CAD build for the part. Positions are in the model's coordinates, mm. A direction names the side the tool comes from. Give positions to 0.01 mm unless a question says otherwise; leave off trailing zeros. Order: outer loops, then holes, each group sorted by start corner. A loop starts at its lowest first (then second) coordinate and runs counter-clockwise, first axis right, second up. Notation, with made-up numbers: M 72.25,36 L 93.25,36 A32 ccw 93.25,72 Z; hole C -1.5,47 d4. An arc over 180 degrees is marked long. Put each result on its own line as item: value. Start each with the question number.
1) Cut at A-A (z = 54). Write the cut outline in (x, y).
2) Drill centre lines: line 1 (Z direction, x = -26.5, y = 5); line 2 (X direction, y = 12.7, z = 102.95); line 3 (Z direction, x = -11.5, y = 13). Where is each one in solid material? Low to high. Write a range as [from, to].
3) Cut at B-B (y = 40). Write the cut outline in (x, z), and give its area (3 significant figures).
4) Tool access for faces 1 (the face through (-27.178, 18, 56)), 2 (the face through (-1.03, 8.05, 75.23)), 3 (the face through (27.178, 31, 102)): list every direction of +Z, -Z, +X, -X, +Y, -Y with a clear straight run to the whole face (end or side of a thin tool).
5) Two-plate mould, pull along X, no slides. Class faces 4 (the face through (0, 16.51, -85)), 5 (the face through (-33.62, 28.93, -55.62)), 6 (the face through (-39.878, 18, -1)): released by +X, released by -X, zero draft, split by the parting line, or undercut.
6) Pin check, flat tips, straight feed: pin 1 (3 mm diameter, centred on x = 32.5, z = 101, fed in from +Y); pin 2 (2 mm diameter, centred on y = 38.5, z = 14.5, fed in from -X); pin 3 (3 mm diameter, centred on x = 4, y = 38.5, fed in from -Z). Stop position of each tip, or through.
7) Cut at C-C (z = -56). Write the cut outline in (x, y).
```python
from build123d import *
from build123d.topology import SkipClean

# Parameters (mm, degrees)
HOUSING_FILLET_LIP_R               = 6.35
UBJ_START                          = 36.068
UBJ_MATERIAL_PREP_DEPTH            = 36.068
UBJ_ARM_TK_DEPTH                   = 79.756
SKETCH32_R                         = 4.5
CAMBERBLOCK_HOLES_DEPTH            = 21.59
SKETCH28_W                         = 54.356
SKETCH28_H                         = 38.9128
UBJ_CROSS_MEMBER_TK_DEPTH          = 5.08
UBJ_MASS_CUTTING_REACH             = 119.247
LBJ_START                          = -36.068
LBJ_MATERIAL_PREP_DEPTH            = 36.068
FLAT_LBJ_PREP_DEPTH                = 10.668
LBJ_SLOT_REACH                     = 117.643
LBJ_WEIGHT_AND_BOLT_CLEARING_REACH = 117.643
LBJ_FILLET_R                       = 6.35
LBJ_HOLE_REACH                     = 221.441
SKETCH14_R                         = 4.7625
MOUTH_WIDEN_DEPTH                  = 125.09324931


with BuildPart() as part:
    # Bearing Sketch → Bearing Revolve (revolve)
    with BuildSketch(Plane(origin=(0, 0, 0), x_dir=(0, 0, -1), z_dir=(1, 0, 0)), mode=Mode.PRIVATE) as bearing_revolve_sk:
        Polygon((-39.878, 0), (-39.878, 48.768), (-32.258, 48.768), (-32.258, 52.578), (-30.99943, 52.578), (-30.99943, 28.194), (-26.289, 28.194), (-26.289, 21.844), (-30.99943, 21.844), (-30.99943, 0), align=None)
    revolve(bearing_revolve_sk.sketch.rotate(Axis((0, 0, 0), (0, 1, 0)), 180), axis=Axis((0, 0, 0), (0, 1, 0)))

    # Housing Fillet Lip
    # the kernel refuses this fillet: 6.35 mm, written as the material it adds along each edge
    with BuildSketch(Plane(origin=(0, 48.768, 0), x_dir=(0, 0, -1), z_dir=(1, 0, 0))) as housing_fillet_lip_piece_1:
        with BuildLine():
            CenterArc((38.077871133, 6.35), HOUSING_FILLET_LIP_R, 203.578178478, 66.421821522)
            Line((32.258, 3.81), (32.141602577, 3.7592))
            ThreePointArc((32.141602577, 3.7592), (32.131, 1.905), (32.131, 0))
            Line((32.131, 0), (32.258, -0.127))
            Line((32.258, -0.127), (38.077871133, -0.127))
            Line((38.077871133, -0.127), (38.077871133, 0))
        make_face()
    revolve(axis=Axis((0, 48.768, 0), (0, 1, 0)))

    # PrepArea(WithadjWidth) → UBJ Material Prep (add)
    with BuildSketch(Plane(origin=(0, 0, 0), x_dir=(1, 0, 0), z_dir=(0, 1, 0)).offset(UBJ_START)):
        with BuildLine():
            Line((-39.878, 0), (-39.878, 46.228))
            Line((-39.878, 46.228), (39.878, 46.228))
            Line((39.878, 46.228), (39.878, 0))
            ThreePointArc((39.878, 0), (0, 39.878), (-39.878, 0))
        make_face()
    extrude(amount=-UBJ_MATERIAL_PREP_DEPTH)

    # Sketch27 → UBJ Arm TK (add)
    with BuildSketch(Plane.ZY.offset(39.878)):
        Polygon((-46.228, 36.068), (-65.278, 21.59), (-104.1908, 21.59), (-104.1908, 0), (-91.959544072, 0), (-46.228, 0), align=None)
    extrude(amount=-UBJ_ARM_TK_DEPTH)

    # Sketch32 → CamberBlock Holes (cut)
    with BuildSketch(Plane(origin=(0, 21.59, 0), x_dir=(1, 0, 0), z_dir=(0, 1, 0))):
        with Locations(Location((-12.7, 84.7344, 0), (0, 0, 270))):
            Circle(SKETCH32_R)
        with Locations(Location((12.7, 84.7344, 0), (0, 0, 270))):
            Circle(SKETCH32_R)
    extrude(amount=-CAMBERBLOCK_HOLES_DEPTH, mode=Mode.SUBTRACT)

    # Sketch28 → UBJ Cross Member TK (cut)
    with BuildSketch(Plane(origin=(0, 21.59, 0), x_dir=(1, 0, 0), z_dir=(0, 1, 0))):
        with Locations((0, 84.7344)):
            Rectangle(SKETCH28_W, SKETCH28_H)
    extrude(amount=-UBJ_CROSS_MEMBER_TK_DEPTH, mode=Mode.SUBTRACT)

    # Sketch30 → UBJ Mass Cutting (cut, up to next)
    with BuildSketch(Plane(origin=(0, 36.068, 0), x_dir=(1, 0, 0), z_dir=(0, 1, 0)), mode=Mode.PRIVATE) as ubj_mass_cutting_sk1:
        with BuildLine():
            Line((-27.178, 65.278), (27.178, 65.278))
            Line((27.178, 65.278), (27.178, 29.182378244))
            ThreePointArc((27.178, 29.182378244), (0, 39.878), (-27.178, 29.182378244))
            Line((-27.178, 29.182378244), (-27.178, 65.278))
        make_face()
    ubj_mass_cutting_tool1 = extrude(ubj_mass_cutting_sk1.sketch, amount=-UBJ_MASS_CUTTING_REACH, mode=Mode.PRIVATE) & part.part
    add(ubj_mass_cutting_tool1.solids().sort_by_distance((0, 36.068, -50.735285))[0], mode=Mode.SUBTRACT)

    # Sketch9 → LBJ Material Prep (add)
    with BuildSketch(Plane.XZ.offset(LBJ_START)):
        with BuildLine():
            Line((-39.878, 0), (-39.878, 105.0925))
            Line((-39.878, 105.0925), (39.878, 105.0925))
            Line((39.878, 105.0925), (39.878, 0))
            ThreePointArc((39.878, 0), (0, 39.878), (-39.878, 0))
        make_face()
    extrude(amount=LBJ_MATERIAL_PREP_DEPTH)

    # Sketch10 → Flat LBJ Prep (cut)
    with SkipClean():  # the faces are left unmerged after this step: merging them gives an invalid solid
        with BuildSketch(Plane(origin=(0, 36.068, 0), x_dir=(1, 0, 0), z_dir=(0, 1, 0))):
            with BuildLine():
                Line((-27.178, -29.182378244), (-27.178, -105.0925))
                Line((-27.178, -105.0925), (27.178, -105.0925))
                Line((27.178, -105.0925), (27.178, -29.182378244))
                ThreePointArc((27.178, -29.182378244), (0, -39.878), (-27.178, -29.182378244))
            make_face()
        extrude(amount=-FLAT_LBJ_PREP_DEPTH, mode=Mode.SUBTRACT)

    # Sketch12 → LBJ Slot (cut, up to next)
    with BuildSketch(Plane(origin=(0, 25.4, 0), x_dir=(1, 0, 0), z_dir=(0, 1, 0)), mode=Mode.PRIVATE) as lbj_slot_sk1:
        with BuildLine():
            Line((-12.7, -78.509539434), (12.7, -78.509539434))
            ThreePointArc((12.7, -78.509539434), (23.0505, -88.860039434), (12.7, -99.210539434))
            Line((12.7, -99.210539434), (-12.7, -99.210539434))
            ThreePointArc((-12.7, -99.210539434), (-23.0505, -88.860039434), (-12.7, -78.509539434))
        make_face()
    lbj_slot_tool1 = extrude(lbj_slot_sk1.sketch, amount=-LBJ_SLOT_REACH, mode=Mode.PRIVATE) & part.part
    add(lbj_slot_tool1.solids().sort_by_distance((0, 25.4, 88.860039))[0], mode=Mode.SUBTRACT)

    # Sketch13 → LBJ Weight and Bolt Clearing (cut, up to next)
    with BuildSketch(Plane(origin=(0, 25.4, 0), x_dir=(1, 0, 0), z_dir=(0, 1, 0)), mode=Mode.PRIVATE) as lbj_weight_and_bolt_clearing_sk1:
        with BuildLine():
            Line((-27.178, -29.182378244), (-27.178, -71.867439434))
            Line((-27.178, -71.867439434), (27.178, -71.867439434))
            Line((27.178, -71.867439434), (27.178, -29.182378244))
            ThreePointArc((27.178, -29.182378244), (0, -39.878), (-27.178, -29.182378244))
        make_face()
    lbj_weight_and_bolt_clearing_tool1 = extrude(lbj_weight_and_bolt_clearing_sk1.sketch, amount=-LBJ_WEIGHT_AND_BOLT_CLEARING_REACH, mode=Mode.PRIVATE) & part.part
    add(lbj_weight_and_bolt_clearing_tool1.solids().sort_by_distance((0, 25.4, 54.061372))[0], mode=Mode.SUBTRACT)

    # LBJ Fillet
    # the kernel refuses this fillet: 6.35 mm, written as the material it adds along each edge
    with BuildSketch(Plane(origin=(-27.178, 25.4, 29.182378244), x_dir=(0.8204405839916299, 0, 0.5717317973835926), z_dir=(0, -1, 0))) as lbj_fillet_piece_1:
        with BuildLine():
            CenterArc((12.120741225, 6.286772968), LBJ_FILLET_R, 145.128922247, 116.778941593)
            Line((6.910943516, 9.917269881), (0, 0))
            ThreePointArc((0, 0), (5.613440626, 0.397065762), (11.226881252, 0))
        make_face()
    extrude(amount=25.4)
    with BuildSketch(Plane(origin=(27.178, 25.4, 29.182378244), x_dir=(-0.8204405839916303, 0, 0.5717317973835919), z_dir=(0, -1, 0))) as lbj_fillet_piece_2:
        with BuildLine():
            CenterArc((12.120741225, -6.286772968), LBJ_FILLET_R, 98.09213616, 116.778941593)
            Line((6.910943516, -9.917269881), (0, 0))
            ThreePointArc((0, 0), (5.613440626, -0.397065762), (11.226881252, 0))
        make_face()
    extrude(amount=25.4)
    with BuildSketch(Plane(origin=(27.178, 25.4, 71.867439434), x_dir=(0, 0, -1), z_dir=(0, -1, 0)), Plane(origin=(-27.178, 25.4, 71.867439434), x_dir=(1, 0, 0), z_dir=(0, -1, 0))) as lbj_fillet_piece_3:
        with BuildLine():
            CenterArc((LBJ_FILLET_R, -LBJ_FILLET_R), LBJ_FILLET_R, 90, 90)
            Line((0, -LBJ_FILLET_R), (0, 0))
            Line((0, 0), (LBJ_FILLET_R, 0))
        make_face()
    extrude(amount=25.4)
    with BuildSketch(Plane(origin=(27.178, 36.068, 29.182378244), x_dir=(-0.8204405839916303, 0, 0.5717317973835919), z_dir=(0, -1, 0))) as lbj_fillet_piece_4:
        with BuildLine():
            CenterArc((12.120741225, -6.286772968), LBJ_FILLET_R, 98.09213616, 116.778941593)
            Line((6.910943516, -9.917269881), (0, 0))
            ThreePointArc((0, 0), (5.613440626, -0.397065762), (11.226881252, 0))
        make_face()
    extrude(amount=10.668)
    with BuildSketch(Plane(origin=(-27.178, 36.068, 29.182378244), x_dir=(0.8204405839916299, 0, 0.5717317973835926), z_dir=(0, -1, 0))) as lbj_fillet_piece_5:
        with BuildLine():
            CenterArc((12.120741225, 6.286772968), LBJ_FILLET_R, 145.128922247, 116.778941593)
            Line((6.910943516, 9.917269881), (0, 0))
            ThreePointArc((0, 0), (5.613440626, 0.397065762), (11.226881252, 0))
        make_face()
    extrude(amount=10.668)

    # LBJ Hole: up to this face of the body (flat: up to its plane)
    lbj_hole_end = Plane(part.part.faces().sort_by_distance((0, 12.7, 71.867439434))[0])
    # Sketch14 → LBJ Hole (cut, up to the picked face)
    with BuildSketch(Plane.XY.offset(105.0925), mode=Mode.PRIVATE) as lbj_hole_sk1:
        with Locations((0, 12.7)):
            Circle(SKETCH14_R)
    lbj_hole_tool1 = split(extrude(lbj_hole_sk1.sketch, amount=-LBJ_HOLE_REACH, mode=Mode.PRIVATE), bisect_by=lbj_hole_end, keep=Keep.BOTH, mode=Mode.PRIVATE)
    add(lbj_hole_tool1.solids().sort_by(Axis((0, 12.7, 105.0925), (0, 0, -1)))[0], mode=Mode.SUBTRACT)

    # Sketch33 → Mouth Widen (cut, through all)
    with BuildSketch(Plane(origin=(0, 0, 0), x_dir=(0, 0, 1), z_dir=(-0.8660254037844398, 0.499999999999998, 0))):
        with BuildLine():
            Line((78.5495, 12.7), (78.5495, 22.86))
            ThreePointArc((78.5495, 22.86), (88.9, 33.2105), (99.2505, 22.86))
            Line((99.2505, 22.86), (99.2505, 12.7))
            ThreePointArc((99.2505, 12.7), (88.9, 2.3495), (78.5495, 12.7))
        make_face()
    mouth_widen = extrude(amount=MOUTH_WIDEN_DEPTH, mode=Mode.SUBTRACT)

    # Mouth Mirror: Mouth Widen across plane
    add(mouth_widen.mirror(Plane(origin=(0, 0, 0), x_dir=(0, 0, 1), z_dir=(1, 0, 0))), mode=Mode.SUBTRACT)


solid = part.part
```
Solution:
1. outline: M -39.88,0 L -27.18,0 L -27.18,36.07 L -39.88,36.07 Z; M 27.18,0 L 39.88,0 L 39.88,36.07 L 27.18,36.07 Z
2. line 1: [-104.19, -65.28], [-29.8, -16.08], [16.08, 38.42], [68.37, 105.09]
2. line 2: [-39.88, -4.76], [4.76, 39.88]
2. line 3: [-104.19, -89.07], [-80.4, -65.28], [-38.18, -28.79], [28.79, 38.18], [71.87, 78.51], [99.21, 105.09]
3. outline: C 0,0 d79.76; hole C 0,0 d62
3. area: 1,980 mm²
4. face 1: +Y
4. face 2: +Z
4. face 3: +Z, +Y
5. face 4: undercut
5. face 5: zero draft
5. face 6: released by -X
6. pin 1: y = 36.07
6. pin 2: x = -37.52
6. pin 3: z = -39.8
7. outline: M -39.88,0 L -27.18,0 L -27.18,28.64 L -39.88,28.64 Z; M 27.18,0 L 39.88,0 L 39.88,28.64 L 27.18,28.64 Z
